Could you check a few things on this model? Use its own coordinates, in mm. Give positions to 0.01 mm unless a question says otherwise; leave off trailing zeros. Loops run counter-clockwise (first coordinate to the right, second up) from the corner with the lowest first, then second, coordinate; pieces in that order, holes last. Notation, with made-up numbers: (37.5, 60) -> (43.5, 60) arc R7 ccw to (43.5, 70) -> close; hole circle Ø3 at (0, 67.25). An arc over 180 degrees is marked (long way). Write item = value, one per line. Start each with the question number.
1) I need wall thicknesses on probe 1 along Z at (x, y) = (-10, 1.95); probe 2 along X at (y, z) = (3.75, 100.5); probe 3 along X at (y, z) = (3.95, -43). Which ranges of each line are inside material? Lowest first, please. Write a range as from..to.
2) I want a section at A-A (z = 83). List the corners of the cut face in (x, y) for me.
3) I want a section at B-B (y = 1). Count the separate pieces of the cut face and the enclosed holes in it, and give its area (3 significant figures).
4) I want a section at C-C (z = -203). List the corners of the cut face in (x, y) for me, and give its area (3 significant figures).
5) I'm going to push flat-ended pins straight in: pin 1 Ø7 at (x, z) = (-49, 55) entering from -Y; pin 2 Ø1 at (y, z) = (2, -132.5) entering from -X. Where does each tip first touch, or does it pass through?
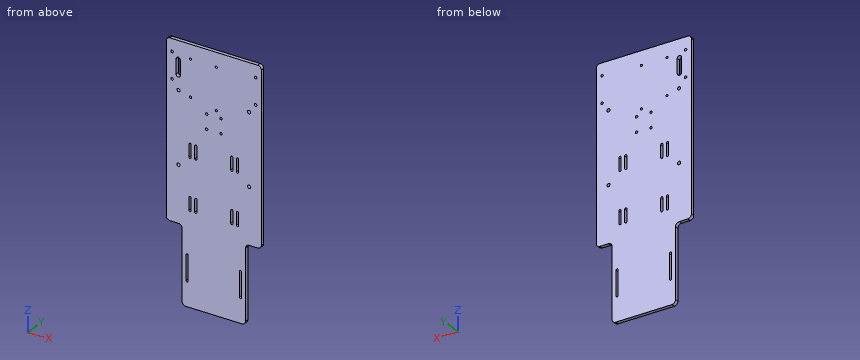
Autodesk Inventor part; units mm, degrees
ref_plane "YZ Plane" through (0, 0, 0) normal (1, 0, 0) x (0, 1, 0)
ref_plane "XZ Plane" through (0, 0, 0) normal (0, 1, 0) x (-1, 0, 0)
ref_plane "XY Plane" through (0, 0, 0) normal (0, 0, 1) x (1, 0, 0)
sketch "Esquisse1" plane through (0, 0, 0) normal (0, 1, 0) x (-1, 0, 0)
  line L0 (66, 120) -> (-66, 120)
  line L1 (-66, 120) -> (-66, -120)
  line L2 (66, -120) -> (66, 120)
  line L3 (66, 120) -> (-66, -120) construction
  line L4 (-66, 120) -> (66, -120) construction
  line L5 (-44, -120) -> (-44, -226)
  line L6 (-44, -226) -> (44, -226)
  line L7 (44, -226) -> (44, -120)
  line L8 (-66, -120) -> (-44, -120)
  line L9 (44, -120) -> (66, -120)
  point P0 (0, 0)
  dimension "d0" = 240
  dimension "d1" = 132
  dimension "d2" = 88
  dimension "d3" = 44
  dimension "d5" = 346
extrude "Extrusion1" add sketch "Esquisse1" along normal blind 5
fillet "Congé1" radius 5 8 edges at (-66, 2.5, 120) (66, 2.5, 120) (66, 2.5, -120) (44, 2.5, -226) (44, 2.5, -120) (-44, 2.5, -226) (-44, 2.5, -120) (-66, 2.5, -120)
sketch "Esquisse3" plane through (0, 5, 0) normal (0, 1, 0) x (1, 0, 0)
  line L0 (-61, -120) -> (61, -120)
  line L1 (-66, 115) -> (-66, -115)
  point P0 (0, 0)
  point P1 (-58, -103)
  dimension "d31" = 17
  dimension "d32" = 8
hole "Perçage2" at (-58, 5, 103) direction (0, -1, 0) diameter 3.5 end through all
pattern_linear "Réseau rectangulaire2" count 2 spacing 36 along (0, 0, -1) count 2 spacing 116 along (1, 0, 0) of "Perçage2"
sketch "Esquisse4" plane through (0, 5, 0) normal (0, 1, 0) x (1, 0, 0)
  line L0 (-49.4, -75) -> (-49.4, -95) construction
  line L1 (-52.4, -75) -> (-52.4, -95)
  line L2 (-46.4, -95) -> (-46.4, -75)
  arc A0 (-46.4, -75) -> (-52.4, -75) centre (-49.4, -75) ccw
  arc A1 (-52.4, -95) -> (-46.4, -95) centre (-49.4, -95) ccw
  line L3 (66, -115) -> (66, 115)
  line L4 (-61, -120) -> (61, -120)
  line L5 (-66, 115) -> (-66, -115)
  point P0 (0, 0)
  point P1 (-49.4, -85)
  dimension "d39" = 3
  dimension "d41" = 35
  dimension "d42" = 20
  dimension "d45" = 16.6
extrude "Extrusion2" cut sketch "Esquisse4" against normal through all
sketch "Esquisse5" plane through (0, 0, 0) normal (0, -1, 0) x (1, 0, 0)
  line L0 (-61, 120) -> (61, 120)
  line L1 (-66, -115) -> (-66, 115)
  point P0 (0, 0)
  point P1 (3.4, 100.5)
  dimension "d53" = 19.5
  dimension "d54" = 69.4
hole "Perçage3" at (3.4, 0, 100.5) direction (0, 1, 0) diameter 3 end through all
pattern_linear "Réseau rectangulaire3" count 2 spacing 57 along (0, 0, -1) of "Perçage3"
sketch "Esquisse6" plane through (0, 0, 0) normal (0, -1, 0) x (1, 0, 0)
  line L0 (-61, 120) -> (61, 120)
  line L1 (-66, -115) -> (-66, 115)
  point P0 (0, 0)
  point P1 (-32.3, 100.5)
  dimension "d65" = 19.5
  dimension "d66" = 33.7
hole "Perçage4" at (-32.3, 0, 100.5) direction (0, 1, 0) diameter 3 end through all
pattern_linear "Réseau rectangulaire4" count 2 spacing 50 along (0, 0, -1) of "Perçage4"
sketch "Esquisse7" plane through (0, 0, 0) normal (0, -1, 0) x (1, 0, 0)
  line L0 (-37, -192) -> (-37, -158) construction
  line L1 (-38.5, -192) -> (-38.5, -158)
  line L2 (-35.5, -158) -> (-35.5, -192)
  arc A0 (-38.5, -192) -> (-35.5, -192) centre (-37, -192) ccw
  arc A1 (-35.5, -158) -> (-38.5, -158) centre (-37, -158) ccw
  line L3 (39, -226) -> (-39, -226)
  line L4 (-44, -221) -> (-44, -125)
  point P0 (0, 0)
  point P1 (-37, -175)
  dimension "d70" = 1.5
  dimension "d71" = 34
  dimension "d72" = 34
  dimension "d73" = 7
extrude "Extrusion3" cut sketch "Esquisse7" against normal through all
mirror "Symétrie1" about plane through (0, 0, 0) normal (1, 0, 0) of "Extrusion3"
sketch "Sketch8" plane through (0, 5, 0) normal (0, 1, 0) x (1, 0, 0)
  line L0 (-61, -120) -> (61, -120) construction
  line L1 (0, -120) -> (0, 226) construction
  line L2 (39, 226) -> (-39, 226) construction
  point P0 (0, 0)
  point P1 (49, -55)
  point P2 (49, 43)
  point P3 (-49, -55)
  point P4 (-49, 43)
  dimension "d86" = 98
  dimension "d89" = 98
  dimension "d92" = 49
  dimension "d93" = 65
hole "Hole5" at (49, 5, 55) at (49, 5, -43) at (-49, 5, 55) at (-49, 5, -43) direction (0, -1, 0) diameter 4.5 end through all
sketch "Sketch9" plane through (0, 5, 0) normal (0, 1, 0) x (1, 0, 0)
  line L0 (25, 11.5) -> (25, 28.5) construction
  line L1 (26.5, 11.5) -> (26.5, 28.5)
  line L2 (23.5, 28.5) -> (23.5, 11.5)
  arc A0 (23.5, 11.5) -> (26.5, 11.5) centre (25, 11.5) ccw
  arc A1 (26.5, 28.5) -> (23.5, 28.5) centre (25, 28.5) ccw
  line L3 (0, 0) -> (47.7976, 0) construction
  line L4 (33, 11.5) -> (33, 28.5) construction
  line L5 (34.5, 11.5) -> (34.5, 28.5)
  line L6 (31.5, 28.5) -> (31.5, 11.5)
  arc A2 (31.5, 11.5) -> (34.5, 11.5) centre (33, 11.5) ccw
  arc A3 (34.5, 28.5) -> (31.5, 28.5) centre (33, 28.5) ccw
  line L7 (0, 0) -> (0, 64.8348) construction
  line L8 (-25, 11.5) -> (-25, 28.5) construction
  line L9 (-33, 11.5) -> (-33, 28.5) construction
  line L10 (-31.5, 11.5) -> (-31.5, 28.5)
  line L11 (-34.5, 28.5) -> (-34.5, 11.5)
  line L12 (-26.5, 28.5) -> (-26.5, 11.5)
  line L13 (-23.5, 11.5) -> (-23.5, 28.5)
  arc A4 (-34.5, 11.5) -> (-31.5, 11.5) centre (-33, 11.5) ccw
  arc A5 (-26.5, 11.5) -> (-23.5, 11.5) centre (-25, 11.5) ccw
  arc A6 (-31.5, 28.5) -> (-34.5, 28.5) centre (-33, 28.5) ccw
  arc A7 (-23.5, 28.5) -> (-26.5, 28.5) centre (-25, 28.5) ccw
  line L14 (33, 81.5) -> (33, 98.5) construction
  line L15 (25, 81.5) -> (25, 98.5) construction
  line L16 (26.5, 81.5) -> (26.5, 98.5)
  line L17 (23.5, 98.5) -> (23.5, 81.5)
  line L18 (31.5, 98.5) -> (31.5, 81.5)
  line L19 (34.5, 81.5) -> (34.5, 98.5)
  arc A8 (23.5, 81.5) -> (26.5, 81.5) centre (25, 81.5) ccw
  arc A9 (31.5, 81.5) -> (34.5, 81.5) centre (33, 81.5) ccw
  arc A10 (26.5, 98.5) -> (23.5, 98.5) centre (25, 98.5) ccw
  arc A11 (34.5, 98.5) -> (31.5, 98.5) centre (33, 98.5) ccw
  line L20 (-25, 81.5) -> (-25, 98.5) construction
  line L21 (-33, 81.5) -> (-33, 98.5) construction
  line L22 (-31.5, 81.5) -> (-31.5, 98.5)
  line L23 (-34.5, 98.5) -> (-34.5, 81.5)
  line L24 (-26.5, 98.5) -> (-26.5, 81.5)
  line L25 (-23.5, 81.5) -> (-23.5, 98.5)
  arc A12 (-34.5, 81.5) -> (-31.5, 81.5) centre (-33, 81.5) ccw
  arc A13 (-26.5, 81.5) -> (-23.5, 81.5) centre (-25, 81.5) ccw
  arc A14 (-31.5, 98.5) -> (-34.5, 98.5) centre (-33, 98.5) ccw
  arc A15 (-23.5, 98.5) -> (-26.5, 98.5) centre (-25, 98.5) ccw
  point P0 (25, 20)
  point P1 (25, 10)
  point P2 (25, 30)
  point P3 (33, 10)
  point P4 (33, 30)
  point P5 (33, 20)
  point P6 (-33, 20)
  point P7 (-25, 20)
  point P8 (-33, 10)
  point P9 (-25, 10)
  point P10 (-33, 30)
  point P11 (-25, 30)
  point P12 (25, 90)
  point P13 (33, 90)
  point P14 (25, 80)
  point P15 (33, 80)
  point P16 (25, 100)
  point P17 (33, 100)
  point P18 (-33, 90)
  point P19 (-25, 90)
  point P20 (-33, 80)
  point P21 (-25, 80)
  point P22 (-33, 100)
  point P23 (-25, 100)
  dimension "d94" = 3
  dimension "d95" = 20
  dimension "d96" = 25
  dimension "d99" = 8
  dimension "d115" = 58
  dimension "d118" = 70
  dimension "d123" = 20
extrude "Extrusion4" cut sketch "Sketch9" against normal through all
sketch "Sketch11" plane through (0, 5, 0) normal (0, 1, 0) x (1, 0, 0)
  line L0 (0, 0) -> (22.9604, 0) construction
  line L1 (22.9604, 0) -> (0, 0) construction
  line L2 (0, 13.4889) -> (0, 0) construction
  point P0 (-10, -35)
  point P1 (10, -35)
  point P2 (-10, -15)
  point P3 (10, -15)
  dimension "d131" = 10
  dimension "d132" = 35
  dimension "d135" = 20
  dimension "d138" = 20
hole "Hole6" at (-10, 5, 35) at (10, 5, 35) at (-10, 5, 15) at (10, 5, 15) direction (0, -1, 0) diameter 3.4 end through all
equation "\"d115\" = 2 * d96 + d99"
properties part number "chassis_3DPrint"
Answer list:
q1.probe_1 = -226..13.3, 16.7..33.3, 36.7..120
q1.probe_2 = -66..-33.8, -30.8..1.9, 4.9..66
q1.probe_3 = -66..-51.25, -46.75..46.75, 51.25..66
q2.outline = (-66, 0) -> (-52.4, 0) -> (-52.4, 5) -> (-66, 5) -> close; (-46.4, 0) -> (66, 0) -> (66, 5) -> (-46.4, 5) -> close
q3.separate_pieces = 1
q3.enclosed_holes = 27
q3.area = 40,000 mm^2
q4.outline = (-44, 0) -> (44, 0) -> (44, 5) -> (-44, 5) -> close
q4.area = 440 mm^2
q5.pin_1 = 0
q5.pin_2 = -44
